```python
from build123d import *

# Parameters (mm, degrees)
RESSALTO_EXTRUS_O1_DEPTH = 49.55
ESBO_O2_W                = 39
ESBO_O2_H                = 26.1
CORTE_EXTRUS_O1_DEPTH    = 8.3
ESBO_O2_3_W              = 0.35
ESBO_O2_3_H              = 26.1
CORTE_EXTRUS_O2_DEPTH    = 40.3
ESBO_O3_W                = 64
ESBO_O3_H                = 4
CORTE_EXTRUS_O3_DEPTH    = 39.3
FILETE2_R                = 5
FILETE3_R                = 10
ESBO_O4_R                = 3
CORTE_EXTRUS_O4_DEPTH    = 90.03983659
CORTE_EXTRUS_O5_DEPTH    = 7.75
ESBO_O6_R                = 1.5
CORTE_EXTRUS_O6_DEPTH    = 10
FILETE4_R                = 4


with BuildPart() as part:
    # Esbo_o1 → Ressalto-extrus_o1 (new body)
    with BuildSketch(Plane(origin=(0, 0, 0), x_dir=(1, 0, 0), z_dir=(0, 1, 0))):
        Polygon((-32, 29.35), (-19.85, 29.35), (-19.85, -25.35), (-32, -25.35), (-32, -33.35), (32, -33.35), (32, -25.35), (19.85, -25.35), (19.85, 29.35), (32, 29.35), (32, 33.35), (-32, 33.35), align=None)
    extrude(amount=RESSALTO_EXTRUS_O1_DEPTH)

    # Esbo_o2 → Corte-extrus_o1 (cut)
    with BuildSketch(Plane(origin=(0, 49.55, 0), x_dir=(1, 0, 0), z_dir=(0, 1, 0))):
        with Locations((0, 16.3)):
            Rectangle(ESBO_O2_W, ESBO_O2_H)
    extrude(amount=-CORTE_EXTRUS_O1_DEPTH, mode=Mode.SUBTRACT)

    # Esbo_o2_3 → Corte-extrus_o2 (cut)
    with BuildSketch(Plane(origin=(0, 49.55, 0), x_dir=(1, 0, 0), z_dir=(0, 1, 0))):
        with Locations((19.675, 16.3)):
            Rectangle(ESBO_O2_3_W, ESBO_O2_3_H)
        with Locations((-19.675, 16.3)):
            Rectangle(ESBO_O2_3_W, ESBO_O2_3_H)
    extrude(amount=-CORTE_EXTRUS_O2_DEPTH, mode=Mode.SUBTRACT)

    # Esbo_o3 → Corte-extrus_o3 (cut)
    with BuildSketch(Plane(origin=(0, 49.55, 0), x_dir=(1, 0, 0), z_dir=(0, 1, 0))):
        with Locations((0, 31.35)):
            Rectangle(ESBO_O3_W, ESBO_O3_H)
    extrude(amount=-CORTE_EXTRUS_O3_DEPTH, mode=Mode.SUBTRACT)

    # Filete2
    filete2_edges = [part.edges().sort_by_distance(p)[0] for p in [
        (-32, 0, -31.35),
        (32, 0, -31.35),
        (-32, 10.25, -31.35),
        (32, 10.25, -31.35),
    ]]
    fillet(filete2_edges, radius=FILETE2_R)

    # Filete3
    filete3_edges = [part.edges().sort_by_distance(p)[0] for p in [
        (0, 41.25, -29.35),
    ]]
    fillet(filete3_edges, radius=FILETE3_R)

    # Esbo_o4 → Corte-extrus_o4 (cut, through all)
    with BuildSketch(Plane(origin=(0, 0, -33.35), x_dir=(-1, 0, 0), z_dir=(0, 0, -1))):
        with Locations((27, 5.25)):
            Circle(ESBO_O4_R)
        with Locations((-27, 5)):
            Circle(ESBO_O4_R)
    extrude(amount=-CORTE_EXTRUS_O4_DEPTH, mode=Mode.SUBTRACT)

    # Esbo_o5 → Corte-extrus_o5 (cut)
    with BuildSketch(Plane(origin=(0, 49.55, 0), x_dir=(1, 0, 0), z_dir=(0, 1, 0))):
        Polygon((-19.85, -4.15), (-19.85, -25.35), (-32, -25.35), (-32, -33.35), (32, -33.35), (32, -25.35), (19.85, -25.35), (19.85, -4.15), align=None)
    extrude(amount=-CORTE_EXTRUS_O5_DEPTH, mode=Mode.SUBTRACT)

    # Esbo_o6 → Corte-extrus_o6 (cut)
    with BuildSketch(Plane(origin=(0, 41.8, 0), x_dir=(1, 0, 0), z_dir=(0, 1, 0))):
        with Locations(Location((17.1, -13.25, 0), (0, 0, 270))):
            Circle(ESBO_O6_R)
        with Locations(Location((-17.1, -13.25, 0), (0, 0, 90))):
            Circle(ESBO_O6_R)
    extrude(amount=-CORTE_EXTRUS_O6_DEPTH, mode=Mode.SUBTRACT)

    # Filete4
    filete4_edges = [part.edges().sort_by_distance(p)[0] for p in [
        (19.5, 20.75, -29.35),
        (19.5, 38.321067812, -26.421067812),
        (-19.5, 38.321067812, -26.421067812),
        (19.5, 41.25, -11.3),
        (-19.5, 41.25, -11.3),
        (-19.5, 20.75, -29.35),
    ]]
    fillet(filete4_edges, radius=FILETE4_R)


solid = part.part
```
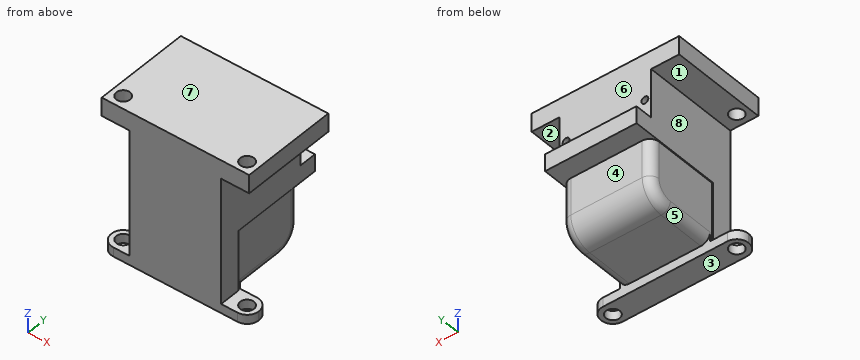
Here's how the part is built. I have some questions about the finished solid (model axes, mm). Face numbers are marked on the shaded views. A direction names the side the tool comes from. Coordinates: 2 decimals unless noted, no trailing zeros. Loops run counter-clockwise (first coordinate to the right, second up) from the corner with the lowest first, then second, coordinate; pieces in that order, holes last. Notation, with made-up numbers: (22, 58.5) -> (59, 58.5) arc R8 ccw to (59, 65.5) -> close; hole circle Ø2 at (10.5, -18). An arc over 180 degrees is marked (long way). Return JSON: item names as keys, results as strings.
1) For the marked faces 1, 2, 3, 4 and 5, which set-ups out of +Z, -Z, +X, -X, +Y, -Y let a thin tool reach every point of the face, with its end or its side?
Results below:
{"face 1": "-X, +Y, -Y", "face 2": "+X, +Y, -Y", "face 3": "-Z, +X, -X, +Y, -Y", "face 4": "-Z, +X, -X, +Y", "face 5": "-Z, -X, +Y"}
2) I need wall thicknesses on line 1 (X direction, y = 37.5, z = 13.25); line 2 (Y direction, x = -27, z = -31); line 3 (Y direction, x = -27, z = 29.5). Which ranges of each line are inside material? Lowest first, please. Write a range as from..to.
Results below:
{"line 1": "-19.85..-18.6, -15.6..15.6, 18.6..19.85", "line 2": "0..2.25, 8.25..10.25", "line 3": "0..2.25, 8.25..41.8"}
3) Thinking about a two-plate mould opening in Z: for the marked faces 6, 7 and 8, which applies, +Z half, -Z half, draft (parallel to the pull), parting line (faces both ways), or undercut?
Results below:
{"face 6": "draft", "face 7": "+Z half", "face 8": "undercut"}
4) If we section it at C-C, the plane x = 10: Write out the boundary of the cut face in (y, z), then the cut area to 3 significant figures.
Results below:
{"outline": "(0, -33.35) -> (10.25, -33.35) -> (10.25, -29.35) -> (31.25, -29.35) arc R10 ccw to (41.25, -19.35) -> (41.25, -3.25) -> (49.55, -3.25) -> (49.55, 4.15) -> (41.8, 4.15) -> (41.8, 33.35) -> (0, 33.35) -> close", "area": "2,680 mm²"}
5) Will these pins go through, and if not, where does the flat tip stop? pin 1 (2.5 mm diameter, centred on x = 17.1, z = 13.25, fed in from -Y); pin 2 (4 mm diameter, centred on x = 2, y = 46.5, fed in from +Z); pin 3 (6 mm diameter, centred on y = 26, z = 0, fed in from +X); pin 4 (8 mm diameter, centred on x = 11, y = 24, fed in from -Z).
Results below:
{"pin 1": "y = 0", "pin 2": "z = 4.15", "pin 3": "x = 19.85", "pin 4": "z = -29.35"}
6) If we section it at D-D, the plane x = 25.5: Write out the boundary of the cut face in (y, z).
Results below:
{"outline": "(0, -33.35) -> (2.4, -33.35) -> (2.4, -29.35) -> (0, -29.35) -> close; (0, 25.35) -> (2.4, 25.35) -> (2.4, 33.35) -> (0, 33.35) -> close; (7.6, -33.35) -> (10.25, -33.35) -> (10.25, -29.35) -> (7.6, -29.35) -> close; (7.6, 25.35) -> (41.8, 25.35) -> (41.8, 33.35) -> (7.6, 33.35) -> close"}
7) If we section it at B-B, the plane x = -21.5: Write out the boundary of the cut face in (y, z).
Results below:
{"outline": "(0, -33.35) -> (10.25, -33.35) -> (10.25, -29.35) -> (0, -29.35) -> close; (0, 25.35) -> (41.8, 25.35) -> (41.8, 33.35) -> (0, 33.35) -> close"}
8) If we section it at A-A, the plane z = 13.25: Write out the boundary of the cut face in (x, y).
Results below:
{"outline": "(-19.85, 0) -> (19.85, 0) -> (19.85, 41.8) -> (18.6, 41.8) -> (18.6, 31.8) -> (15.6, 31.8) -> (15.6, 41.8) -> (-15.6, 41.8) -> (-15.6, 31.8) -> (-18.6, 31.8) -> (-18.6, 41.8) -> (-19.85, 41.8) -> close"}
